from build123d import *

# Parameters (mm, degrees)
MODEL_R                 = 1.5
SALIENTE_EXTRUIR1_DEPTH = 3


with BuildPart() as part:
    # Model → Saliente-Extruir1 (new body)
    with BuildSketch(Plane.XY):
        with BuildLine():
            Line((198.613156537, 287.328333228), (193.181176022, 287.328333228))
            Line((193.181176022, 287.328333228), (184.260234476, 290.817294259))
            Line((184.260234476, 290.817294259), (163.611370869, 311.466157866))
            ThreePointArc((163.611370869, 311.466157866), (162.151465799, 312.441635247), (160.429390353, 312.784177351))
            Line((160.429390353, 312.784177351), (147.730106437, 312.825505508))
            Line((147.730106437, 312.825505508), (147.701468292, 312.825598707))
            ThreePointArc((147.701468292, 312.825598707), (146.01766119, 312.49066865), (144.590198455, 311.536868544))
            Line((144.590198455, 311.536868544), (144.448777098, 311.395447188))
            ThreePointArc((144.448777098, 311.395447188), (143.160046936, 308.284177351), (144.448777098, 305.172907513))
            Line((144.448777098, 305.172907513), (169.975331899, 279.646352713))
            ThreePointArc((169.975331899, 279.646352713), (171.435236969, 278.670875332), (173.157312415, 278.328333228))
            Line((173.157312415, 278.328333228), (198.613156537, 278.328333228))
            ThreePointArc((198.613156537, 278.328333228), (203.113156537, 282.828333228), (198.613156537, 287.328333228))
        make_face()
        with Locations((166.793351384, 289.192294259)):
            Circle(MODEL_R, mode=Mode.SUBTRACT)
        with Locations((160.429390353, 295.556255289)):
            Circle(MODEL_R, mode=Mode.SUBTRACT)
        with Locations((173.157312415, 282.828333228)):
            Circle(MODEL_R, mode=Mode.SUBTRACT)
        with Locations((185.885234476, 282.828333228)):
            Circle(MODEL_R, mode=Mode.SUBTRACT)
        with Locations((198.613156537, 282.828333228)):
            Circle(MODEL_R, mode=Mode.SUBTRACT)
        with Locations((179.521273445, 289.192294259)):
            Circle(MODEL_R, mode=Mode.SUBTRACT)
        with Locations((173.157312415, 295.556255289)):
            Circle(MODEL_R, mode=Mode.SUBTRACT)
        with Locations((154.065429323, 301.92021632)):
            Circle(MODEL_R, mode=Mode.SUBTRACT)
        with Locations((166.793351384, 301.92021632)):
            Circle(MODEL_R, mode=Mode.SUBTRACT)
        with Locations((147.701468292, 308.284177351)):
            Circle(MODEL_R, mode=Mode.SUBTRACT)
        with Locations((160.429390353, 308.284177351)):
            Circle(MODEL_R, mode=Mode.SUBTRACT)
    extrude(amount=SALIENTE_EXTRUIR1_DEPTH)


solid = part.part
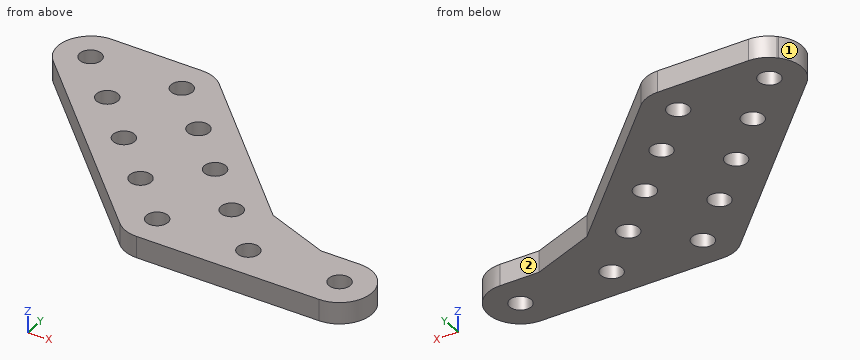
Verification items for the finished model (mm, model axes). Face numbers are marked on the shaded views. A direction names the side the tool comes from. Round coordinates to 2 decimals unless told otherwise and drop trailing zeros. Loops run counter-clockwise (first coordinate to the right, second up) from the corner with the lowest first, then second, coordinate; pieces in that order, holes last. Notation, with made-up numbers: (57, 10.25) - (106, 10.25) arc R10 cw to (106, 22.25) - close; hole circle Ø9 at (-1, 38.5). An arc over 180 degrees is marked (long way). Use a Markdown table: item, result. Add a question column.
1. Thickness scan on probe 1 along X at (y, z) = (294.5, 0.2); probe 2 along X at (y, z) = (284, 0.9); probe 3 along X at (y, z) = (307, 0.9). Record the ranges inside material, lowest first. Write a range as [from, to].
2. Section check C-C, the plane x = 172.5. Record the boundary of the cut face in (y, z).
3. Access from +Z, -Z, +X, -X, +Y, -Y to the whole of each face (thin tool, end or side, straight path). Record for the marked faces 1 and 2.
4. Section check B-B, the plane y = 309. Record the boundary of the cut face in (x, z).
5. Gauge pin test, flat end, axial feed: pin 1 (4 mm diameter, centred on x = 147.7, y = 308.28, fed in from +Z). Record the tip position at first contact, or that the pin passes through.
6. Section check D-D, the plane x = 196. Record the boundary of the cut face in (y, z).
7. Section check A-A, the plane z = 2.25. Give the number of separate pieces and of enclosed holes in the cut face, plus the area to 3 significant figures.
Checks:
| question | item | result |
|---|---|---|
| 1 | probe 1 | x = [155.12, 159.36], [161.49, 172.09], [174.22, 180.58] |
| 1 | probe 2 | x = [165.62, 172.22], [174.09, 184.95], [186.82, 197.68], [199.55, 202.96] |
| 1 | probe 3 | x = [143.35, 146.93], [148.48, 159.65], [161.2, 168.08] |
| 2 | outline | (278.38, 0) - (281.48, 0) - (281.48, 3) - (278.38, 3) - close; (284.18, 0) - (294.21, 0) - (294.21, 3) - (284.18, 3) - close; (296.9, 0) - (302.58, 0) - (302.58, 3) - (296.9, 3) - close |
| 3 | face 1 | +Z, -Z, -X |
| 3 | face 2 | +Z, -Z, +X, +Y |
| 4 | outline | (143.22, 0) - (146.38, 0) - (146.38, 3) - (143.22, 3) - close; (149.02, 0) - (159.11, 0) - (159.11, 3) - (149.02, 3) - close; (161.75, 0) - (166.08, 0) - (166.08, 3) - (161.75, 3) - close |
| 5 | pin 1 | stops at z = 3 |
| 6 | outline | (278.33, 0) - (287.33, 0) - (287.33, 3) - (278.33, 3) - close |
| 7 | separate pieces | 1 |
| 7 | enclosed holes | 11 |
| 7 | area | 873 mm^2 |
